Could you check a few things on this model? Use its own coordinates, in mm. A direction names the side the tool comes from. Give positions to 0.01 mm unless a question says otherwise; leave off trailing zeros. Order: outer loops, then holes, each group sorted by start corner. A loop starts at its lowest first (then second) coordinate and runs counter-clockwise, first axis right, second up. Notation, with made-up numbers: (33.5, 86.25) -> (56.5, 86.25) arc R9 ccw to (56.5, 102.25) -> close; hole circle Ø9 at (52, 20.5). An arc over 180 degrees is marked (long way). One line per item, written item: value.
```python
from build123d import *

# Parameters (mm, degrees)
SKETCH1_W                = 214.089522673
SKETCH1_H                = 271.033566845
BOSS_EXTRUDE1_DEPTH      = 10
SKETCH3_W                = 107.044761337
SKETCH3_H                = 271.033566845
CUT_EXTRUDE1_DEPTH       = 252.253590179
CUT_EXTRUDE2_DEPTH       = 249.55642867
BOSS_EXTRUDE3_DEPTH      = 40
CUT_EXTRUDE3_START       = -165.689856025
CUT_EXTRUDE3_DEPTH       = 205.862728092
CUT_EXTRUDE4_DEPTH       = 250.960593361
CUT_EXTRUDE5_DEPTH       = 250.960593361
BOSS_EXTRUDE5_DEPTH      = 45
CUT_EXTRUDE7_DEPTH       = 253.784190336
CUT_EXTRUDE9_DEPTH       = 253.784190336
CUT_EXTRUDE10_DEPTH      = 105
BOSS_EXTRUDE6_DEPTH      = 13.546139965
BOSS_EXTRUDE7_DEPTH      = 30
CUT_EXTRUDE12_DEPTH      = 30
SKETCH30_W               = 11.3
SKETCH30_H               = 54
CUT_EXTRUDE13_DEPTH      = 30
CUT_EXTRUDE14_DEPTH      = 30
CUT_EXTRUDE14_DEPTH_BACK = 101.665148292
SKETCH31_W               = 44.683801498
SKETCH31_H               = 21.311404518


with BuildPart() as part:
    # Sketch1 → Boss-Extrude1 (new body)
    with BuildSketch(Plane(origin=(0, 0, 0), x_dir=(1, 0, 0), z_dir=(0, 1, 0))):
        with Locations((-3.148375333, -90.062114546)):
            Rectangle(SKETCH1_W, SKETCH1_H)
    extrude(amount=BOSS_EXTRUDE1_DEPTH)

    # Sketch3 → Cut-Extrude1 (cut, through all)
    with BuildSketch(Plane(origin=(0, 10, 0), x_dir=(1, 0, 0), z_dir=(0, 1, 0))):
        with Locations((-56.670756002, -90.062114546)):
            Rectangle(SKETCH3_W, SKETCH3_H)
    extrude(amount=-CUT_EXTRUDE1_DEPTH, mode=Mode.SUBTRACT)

    # Sketch4 → Cut-Extrude2 (cut, through all)
    with BuildSketch(Plane(origin=(0, 10, 0), x_dir=(1, 0, 0), z_dir=(0, 1, 0))):
        Polygon((103.896386003, -181.239506042), (100.834918545, -173.848469781), (9.996584241, 45.454668877), (103.896386003, 45.454668877), align=None)
    extrude(amount=-CUT_EXTRUDE2_DEPTH, mode=Mode.SUBTRACT)

    # Sketch6 → Boss-Extrude3 (add, along a direction that is not the sketch's normal)
    with BuildSketch(Plane(origin=(0, 10, 0), x_dir=(1, 0, 0), z_dir=(0, 1, 0))):
        Polygon((99.572063218, -170.799667324), (103.896386003, -181.239506042), (-3.148375333, -225.578897968), (-3.148375333, -213.347866105), align=None)
    extrude(amount=BOSS_EXTRUDE3_DEPTH, dir=(-0.2705980500730979, 0.7071067811865489, -0.6532814824381872))

    # Cut-Extrude3: read off the stored shape, not the designer's step
    # Cut-Extrude3 outline → Cut-Extrude3 (cut)
    with BuildSketch(Plane(origin=(0, 0, 0), x_dir=(1, 0, 0), z_dir=(0, 0.6785983445458481, -0.7345095552677544)).offset(CUT_EXTRUDE3_START)):
        Polygon((-3.148375333, -165), (-3.148375333, -152.122604304), (-13.972297336, -155.165042499), (-15, -155.45391393), (-15, -165), align=None)
    extrude(amount=CUT_EXTRUDE3_DEPTH, mode=Mode.SUBTRACT)

    # Sketch8 → Cut-Extrude4 (cut, through all)
    with BuildSketch(Plane(origin=(0, 10, 0), x_dir=(1, 0, 0), z_dir=(0, 1, 0))):
        Polygon((-3.148375333, -225.578897968), (103.896386003, -181.239506042), (103.896386003, -225.578897968), align=None)
    extrude(amount=-CUT_EXTRUDE4_DEPTH, mode=Mode.SUBTRACT)

    # Sketch9 → Cut-Extrude5 (cut, through all)
    with BuildSketch(Plane(origin=(0, 10, 0), x_dir=(1, 0, 0), z_dir=(0, 1, 0))):
        Polygon((-3.148375333, -213.347866105), (99.572063218, -170.799667324), (9.996584241, 45.454668877), (-3.148375333, 45.454668877), align=None)
    extrude(amount=-CUT_EXTRUDE5_DEPTH, mode=Mode.SUBTRACT)

    # Sketch13 → Boss-Extrude5 (add)
    with BuildSketch(Plane.XZ):
        Polygon((-3.148375333, 225.578897968), (-3.148375333, 213.347866105), (99.572063218, 170.799667324), (103.896386003, 181.239506042), align=None)
    extrude(amount=BOSS_EXTRUDE5_DEPTH)

    # Sketch14 → Cut-Extrude7 (cut, through all)
    with BuildSketch(Plane(origin=(24.603270673, 0, -10.191008392), x_dir=(-0.38268343236508967, 0, -0.9238795325112868), z_dir=(0.9238795325112867, 0, -0.3826834323650896))):
        Polygon((-178.918624473, 38.284271247), (-173.268624473, 32.634271247), (-167.618624473, 38.284271247), align=None)
    extrude(amount=-CUT_EXTRUDE7_DEPTH, mode=Mode.SUBTRACT)

    # Sketch21 → Cut-Extrude9 (cut, through all)
    with BuildSketch(Plane(origin=(24.603270673, 0, -10.191008392), x_dir=(-0.38268343236508967, 0, -0.9238795325112868), z_dir=(0.9238795325112867, 0, -0.3826834323650896))):
        Polygon((-178.918624473, 38.284271247), (-173.268624473, 32.634271247), (-186.710507565, 19.192388155), (-188.372208501, 20.854089091), (-197.564596656, 11.661700936), (-199.891194785, 13.988299064), (-190.698806629, 23.18068722), (-192.360507565, 24.842388155), align=None)
    extrude(amount=-CUT_EXTRUDE9_DEPTH, mode=Mode.SUBTRACT)

    # Sketch26 → Cut-Extrude10 (cut)
    with BuildSketch(Plane(origin=(24.603270673, 0, -10.191008392), x_dir=(-0.38268343236508967, 0, -0.9238795325112868), z_dir=(0.9238795325112867, 0, -0.3826834323650896))):
        Polygon((-195.90289572, 9), (-195.90289572, -45), (-207.20289572, -45), (-207.20289572, 9), (-204.80289572, 9), (-204.80289572, 11.1), (-202.60289572, 11.1), (-202.60289572, 9), (-200.50289572, 9), (-200.50289572, 11.1), (-198.30289572, 11.1), (-198.30289572, 9), align=None)
    extrude(amount=-CUT_EXTRUDE10_DEPTH, mode=Mode.SUBTRACT)

    # Sketch27 → Boss-Extrude6 (add, along a direction that is not the sketch's normal)
    with BuildSketch(Plane(origin=(35.57097911, -92.95144786, 85.875940195), x_dir=(0.9626924198811571, 0.19875685341551327, -0.18362738881693624), z_dir=(-0.2705980500730966, 0.7071067811865525, -0.6532814824381838))):
        Polygon((-40.219860097, -165.940754997), (-39.260177115, -165.659670359), (-38.335322468, -168.817321636), (-40.219860097, -169.369289928), align=None)
    extrude(amount=BOSS_EXTRUDE6_DEPTH, dir=(0, 0.6785983445458494, -0.7345095552677533))

    # Sketch28 → Boss-Extrude7 (add, along a direction that is not the sketch's normal)
    with BuildSketch(Plane(origin=(32.053204459, -83.759059705, 77.383280924), x_dir=(0.9626924198811573, 0.1987568534155131, -0.18362738881693524), z_dir=(-0.27059805007309584, 0.7071067811865541, -0.6532814824381823))):
        Polygon((-23.130198055, -160.935308873), (-23.790746954, -158.680053865), (-36.565759807, -162.4217685), (-36.565759807, -170.747754034), (-21.54479451, -166.348215158), (-22.205343409, -164.09296015), (-34.681222178, -167.74706044), (-35.606076824, -164.589409163), align=None)
    extrude(amount=BOSS_EXTRUDE7_DEPTH, dir=(0, 0.6785983445458483, -0.7345095552677544))

    # Sketch29 → Cut-Extrude12 (cut)
    with BuildSketch(Plane(origin=(41.559974827, 108.60144786, 100.334654879), x_dir=(0.9626924198811563, -0.1987568534155138, -0.18362738881693985), z_dir=(0.2705980500730995, 0.7071067811865461, 0.6532814824381895))):
        Polygon((-46.440949609, -107.03174708), (-31.419984312, -107.03174708), (-31.419984312, -102.632208204), align=None)
    extrude(amount=-CUT_EXTRUDE12_DEPTH, mode=Mode.SUBTRACT)

    # Sketch30 → Cut-Extrude13 (cut)
    with BuildSketch(Plane(origin=(-72.40408024, 0, 29.990752007), x_dir=(-0.3826834323650857, 0, -0.9238795325112884), z_dir=(0.9238795325112884, 0, -0.3826834323650857))):
        with Locations((-201.55289572, -18)):
            Rectangle(SKETCH30_W, SKETCH30_H)
    extrude(amount=-CUT_EXTRUDE13_DEPTH, mode=Mode.SUBTRACT)

    # Sketch31 → Cut-Extrude14 (cut, two sides: drawn at the far end of the back side and taken through both)
    with BuildSketch(Plane(origin=(74.968792545, 0, 180.990675716), x_dir=(-0.9238795325112865, 0, 0.38268343236509056), z_dir=(-0.38268343236509056, 0, -0.9238795325112865)).offset(-CUT_EXTRUDE14_DEPTH_BACK)):
        with Locations((-4.288487529, 19.655702259)):
            Rectangle(SKETCH31_W, SKETCH31_H)
    extrude(amount=CUT_EXTRUDE14_DEPTH + CUT_EXTRUDE14_DEPTH_BACK, mode=Mode.SUBTRACT)

    # Mirror4: part across plane


with BuildPart() as part_1:
    add(part.part)
    add(part.part.mirror(Plane(origin=(-3.148375333, 0, 225.578897968), x_dir=(0, 0, 1), z_dir=(1, 0, 0))))


solid = part_1.part
```
1) Suppose I cut it at A-A, the plane y = 35. Write out the boundary of the cut face in (x, z), then the cut area to 3 significant figures.
Answer below:
outline: (-17.61, 192.53) -> (-16.97, 189.2) -> (-4.96, 194.17) -> (-4.07, 189.5) -> (-16.08, 184.53) -> (-15.45, 181.19) -> (-3.15, 186.29) -> (9.15, 181.19) -> (9.79, 184.53) -> (-2.22, 189.5) -> (-1.33, 194.17) -> (10.68, 189.2) -> (11.31, 192.53) -> (-3.15, 198.52) -> close
area: 206 mm2
2) Suppose I cut it at D-D, the plane x = 0. Write out the boundary of the cut face in (y, z), then the cut area to 3 significant figures.
Answer below:
outline: (9, 212.04) -> (10, 212.04) -> (38.45, 181.25) -> (40.25, 182.9) -> (11.66, 213.84) -> (13.99, 216.36) -> (42.76, 185.22) -> (44.55, 186.88) -> (10, 224.27) -> (9, 224.27) -> close
area: 253 mm2
3) If I drill on line 1 along Z through (x, y) = (43, 11); line 2 along Z through (x, y) = (-17, 11); line 3 along Z through (x, y) = (27, 19.5), over which ranges is the centre line in solid material (lowest first)?
Answer below:
line 1: z = 193.15 to 196.83, 199.21 to 201.48, 203.87 to 205.38
line 2: z = 206.53 to 210.21, 212.59 to 214.86, 217.24 to 218.76
line 3: z = 191.24 to 194.17, 199.21 to 202.81
4) For P1, Ø1.5, axis at x = -0.5, z = 205, coming from the +Y side; P2, Ø8, axis at x = 44.5, z = 209.5, coming from the -Y side; P3, Ø1, axis at x = -15, z = 185, coming from the -Y side; P4, Ø1.5, axis at x = -43, z = 209, coming from the +Y side, each with a flat end and sliding along its axis, tell me the tip position at first contact or that it passes through.
Answer below:
P1: stops at y = 28.75
P2: stops at y = 9
P3: stops at y = 31.15
P4: stops at y = 10.82
5) We'd pull the mould along Z, two halves only. Please class faces 1 (the flat face through (34, 11.1, 206)), 2 (the flat face through (30.19, 9.51, 211.77)), 3 (the flat face through (-40.417, 24, 193.165)): +Z half, -Z half, draft (parallel to the pull), parting line (faces both ways), or undercut.
Answer below:
face 1: undercut
face 2: +Z half
face 3: -Z half
6) Suppose I cut it at C-C, the plane z = 223.5. Write out the boundary of the cut face in (x, y).
Answer below:
outline: (-8.17, 9) -> (1.87, 9) -> (1.87, 10) -> (-3.15, 11.92) -> (-8.17, 10) -> close
7) Suppose I cut it at B-B, the plane x = -54. Write out the boundary of the cut face in (y, z), then the cut area to 3 significant figures.
Answer below:
outline: (9, 192.28) -> (10, 192.28) -> (19.19, 182.33) -> (20.85, 184.13) -> (11.66, 194.08) -> (13.99, 196.6) -> (23.18, 186.65) -> (24.84, 188.45) -> (10, 204.52) -> (9, 204.52) -> (9, 201.92) -> (11.1, 201.92) -> (11.1, 199.54) -> (9, 199.54) -> (9, 197.26) -> (11.1, 197.26) -> (11.1, 194.88) -> (9, 194.88) -> close
area: 103 mm2
8) For faces 4 (the flat face through (31.736, 10.065, 201.496)), 5 (the flat face through (27.14, 9.51, 200.8)), 6 (the flat face through (-36.49, 9.51, 211.77)), which set-ups out of +Z, -Z, +X, -X, +Y, -Y let a thin tool reach every point of the face, with its end or its side?
Answer below:
face 4: -Y
face 5: -Z, -Y
face 6: +Z, -X, +Y, -Y
